from build123d import *

# Parameters (mm, degrees)
F0_W      = 63.5
F0_H      = 63.5
F1_DEPTH  = 3.175
F1_FACE_W = 63.5
F1_FACE_H = 63.5
F2_DEPTH  = 3.175
F3_R      = 12.7
F4_DEPTH  = 6.35
F5_DEPTH  = 25.4
F6_DEPTH  = 25.4
F7_DEPTH  = 25.4
F8_DEPTH  = 25.4


with BuildPart() as f1:
    # F0 (on Top) → F1 (new body)
    with BuildSketch(Plane.XY):
        Rectangle(F0_W, F0_H)
    extrude(amount=F1_DEPTH)

    # F1_face (on face) → F2 (join)
    with BuildSketch(Plane(origin=(0, 0, 0), x_dir=(1, 0, 0), z_dir=(0, 0, -1))):
        Rectangle(F1_FACE_W, F1_FACE_H)
    extrude(amount=F2_DEPTH)

    # F3 (on face) → F4 (cut)
    with BuildSketch(Plane.XY.offset(3.175)):
        Circle(F3_R)
        Polygon((0.889, 31.75), (0, 31.75), (-0.889, 31.75), (-0.889, 25.4), (0.889, 25.4), align=None)
        Polygon((31.75, -0.889), (31.75, 0), (31.75, 0.889), (25.4, 0.889), (25.4, -0.889), align=None)
        Polygon((-0.889, -31.75), (0, -31.75), (0.889, -31.75), (0.889, -25.4), (-0.889, -25.4), align=None)
        Polygon((-31.75, 0.889), (-31.75, 0), (-31.75, -0.889), (-25.4, -0.889), (-25.4, 0.889), align=None)
    extrude(amount=-F4_DEPTH, mode=Mode.SUBTRACT)

    # F3 (on face) → F5 (cut)
    with BuildSketch(Plane.XY.offset(3.175)):
        Circle(F3_R)
        Polygon((0.889, 31.75), (0, 31.75), (-0.889, 31.75), (-0.889, 25.4), (0.889, 25.4), align=None)
        Polygon((31.75, -0.889), (31.75, 0), (31.75, 0.889), (25.4, 0.889), (25.4, -0.889), align=None)
        Polygon((-0.889, -31.75), (0, -31.75), (0.889, -31.75), (0.889, -25.4), (-0.889, -25.4), align=None)
        Polygon((-31.75, 0.889), (-31.75, 0), (-31.75, -0.889), (-25.4, -0.889), (-25.4, 0.889), align=None)
    extrude(amount=-F5_DEPTH, mode=Mode.SUBTRACT)

    # F3 (on face) → F6 (cut)
    with BuildSketch(Plane.XY.offset(3.175)):
        Circle(F3_R)
        Polygon((0.889, 31.75), (0, 31.75), (-0.889, 31.75), (-0.889, 25.4), (0.889, 25.4), align=None)
        Polygon((31.75, -0.889), (31.75, 0), (31.75, 0.889), (25.4, 0.889), (25.4, -0.889), align=None)
        Polygon((-0.889, -31.75), (0, -31.75), (0.889, -31.75), (0.889, -25.4), (-0.889, -25.4), align=None)
        Polygon((-31.75, 0.889), (-31.75, 0), (-31.75, -0.889), (-25.4, -0.889), (-25.4, 0.889), align=None)
    extrude(amount=-F6_DEPTH, mode=Mode.SUBTRACT)

    # F3 (on face) → F7 (cut)
    with BuildSketch(Plane.XY.offset(3.175)):
        Circle(F3_R)
        Polygon((0.889, 31.75), (0, 31.75), (-0.889, 31.75), (-0.889, 25.4), (0.889, 25.4), align=None)
        Polygon((31.75, -0.889), (31.75, 0), (31.75, 0.889), (25.4, 0.889), (25.4, -0.889), align=None)
        Polygon((-0.889, -31.75), (0, -31.75), (0.889, -31.75), (0.889, -25.4), (-0.889, -25.4), align=None)
        Polygon((-31.75, 0.889), (-31.75, 0), (-31.75, -0.889), (-25.4, -0.889), (-25.4, 0.889), align=None)
    extrude(amount=-F7_DEPTH, mode=Mode.SUBTRACT)

    # F3 (on face) → F8 (cut)
    with BuildSketch(Plane.XY.offset(3.175)):
        Circle(F3_R)
        Polygon((0.889, 31.75), (0, 31.75), (-0.889, 31.75), (-0.889, 25.4), (0.889, 25.4), align=None)
        Polygon((31.75, -0.889), (31.75, 0), (31.75, 0.889), (25.4, 0.889), (25.4, -0.889), align=None)
        Polygon((-0.889, -31.75), (0, -31.75), (0.889, -31.75), (0.889, -25.4), (-0.889, -25.4), align=None)
        Polygon((-31.75, 0.889), (-31.75, 0), (-31.75, -0.889), (-25.4, -0.889), (-25.4, 0.889), align=None)
    extrude(amount=-F8_DEPTH, mode=Mode.SUBTRACT)


solid = f1.part
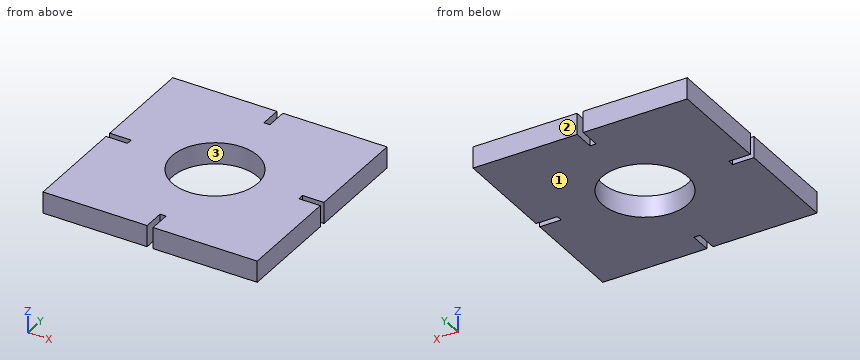
CAD build for the part. Positions are in the model's coordinates, mm. Face numbers are marked on the shaded views. Coordinates: 2 decimals unless noted, no trailing zeros. Loops run counter-clockwise (first coordinate to the right, second up) from the corner with the lowest first, then second, coordinate; pieces in that order, holes last. Notation, with made-up numbers: (-20, 46) - (-5, 46) arc R18 ccw to (-5, 77) - close; hole circle Ø7 at (65, 23.25). An arc over 180 degrees is marked (long way). Use one line per item in the form item = value. Start each with the question number.
1) Band-saw the part on C-C (z = -1.5). Give the cut face in (x, y), and give its area (3 significant figures).
2) Flat gauge pins, fed straight in: pin 1 (0.5 mm diameter, centred on y = -0.5, z = 0.5, fed in from +X); pin 2 (0.5 mm diameter, centred on x = 0, z = 0, fed in from -Y); pin 3 (1.4 mm diameter, centred on y = 0, z = -1, fed in from -X). Where does each tip first touch, or does it go through?
3) Band-saw the part on B-B (y = 0). Give the cut face in (x, z) (3 decimals), and give its area (3 significant figures).
4) Band-saw the part on A-A (x = -28). Give the cut face in (y, z) (3 decimals), and give its area (3 significant figures).
5) Drill centre lines: L1, parallel to Y at x = 0, z = 1.5; L2, parallel to X at y = 1.5, z = -0.75; L3, parallel to Y at x = 8, z = -0.5. Where is each one in solid material? Low to high. Write a range as from..to.
6) Two-plate mould, pull along Y, no slides. Class the marked faces 1, 2 and 3: +Y half, -Y half, draft (parallel to the pull), parting line (faces both ways), or undercut.
Check values:
q1.outline = (-31.75, -31.75) - (-0.89, -31.75) - (-0.89, -25.4) - (0.89, -25.4) - (0.89, -31.75) - (31.75, -31.75) - (31.75, -0.89) - (25.4, -0.89) - (25.4, 0.89) - (31.75, 0.89) - (31.75, 31.75) - (0.89, 31.75) - (0.89, 25.4) - (-0.89, 25.4) - (-0.89, 31.75) - (-31.75, 31.75) - (-31.75, 0.89) - (-25.4, 0.89) - (-25.4, -0.89) - (-31.75, -0.89) - close; hole circle Ø25.4 at (0, 0)
q1.area = 3,480 mm2
q2.pin_1 = 25.4
q2.pin_2 = -25.4
q2.pin_3 = -25.4
q3.outline = (-25.4, -3.175) - (-12.7, -3.175) - (-12.7, 3.175) - (-25.4, 3.175) - close; (12.7, -3.175) - (25.4, -3.175) - (25.4, 3.175) - (12.7, 3.175) - close
q3.area = 161 mm2
q4.outline = (-31.75, -3.175) - (-0.889, -3.175) - (-0.889, 3.175) - (-31.75, 3.175) - close; (0.889, -3.175) - (31.75, -3.175) - (31.75, 3.175) - (0.889, 3.175) - close
q4.area = 392 mm2
q5.L1 = -25.4..-12.7, 12.7..25.4
q5.L2 = -31.75..-12.61, 12.61..31.75
q5.L3 = -31.75..-9.86, 9.86..31.75
q6.face_1 = draft
q6.face_2 = +Y half
q6.face_3 = undercut
